```python
from build123d import *

# Parameters (mm, degrees)
PAD_DEPTH    = 25
POCKET_DEPTH = 5
FILLET_R     = 1


with BuildPart() as part:
    # Sketch → Pad (new body)
    with BuildSketch(Plane.XY):
        with BuildLine():
            Line((-6.8, 40), (-6.8, 0))
            Line((-6.8, 0), (-5.8, 0))
            ThreePointArc((-5.8, 0), (-4.679209, 3.420545), (-4.3, 7))
            Line((-4.3, 7), (-4.3, 37))
            ThreePointArc((-2.5, 37), (-3.4, 37.9), (-4.3, 37))
            Line((-2.5, 37), (-2.5, 6.999997))
            ThreePointArc((-2.5, 6.999997), (-1.632155, 3.363514), (0, 0))
            Line((0, 0), (0, 40))
            ThreePointArc((0, 40), (-3.4, 43.4), (-6.8, 40))
        make_face()
    extrude(amount=PAD_DEPTH)

    # Sketch001 → Pocket (cut)
    with BuildSketch(Plane(origin=(-7.5, 0, 0), x_dir=(0, -1, 0), z_dir=(-1, 0, 0))):
        with BuildLine():
            ThreePointArc((-12.608682, 0), (-0.108682, 12.5), (-12.608682, 25))
            Line((-12.608682, 25), (7.391318, 25))
            Line((7.391318, 25), (7.391318, 0))
            Line((7.391318, 0), (-12.608682, 0))
        make_face()
    extrude(amount=-POCKET_DEPTH, mode=Mode.SUBTRACT)

    # Fillet
    fillet_edges = [part.edges().sort_by_distance(p)[0] for p in [
        (-6.8, 26.304341, 0),
        (-6.8, 0.108682, 12.5),
        (-6.8, 26.304341, 25),
        (-6.8, 40, 12.5),
    ]]
    fillet(fillet_edges, radius=FILLET_R)


solid = part.part
```
Input: part model. Units: mm. Frame: model coordinates. A direction names the side the tool comes from. Round coordinates to 2 decimals unless told otherwise and drop trailing zeros. Loops run counter-clockwise (first coordinate to the right, second up) from the corner with the lowest first, then second, coordinate; pieces in that order, holes last.
1) Set-up query: faces 5 (the cylindrical face through (-5.56, 0.96, 7.97)), 6 (the flat face through (-4.3, 22, 12)), 7 (the cylindrical face through (-6.515, 26.496, 24.699)). Return all of +Z, -Z, +X, -X, +Y, -Y with unobstructed straight access to the full face (end or side cutting, diameter ignored); none if empty.
Ans:
face 5: -X, -Y
face 6: +Z, -Z, -Y
face 7: +Z, -X, +Y, -Y
2) Pull-direction query (X, two-part tool) for faces 1 (the cylindrical face through (-1.65, 3.41, 12.32)), 2 (the flat face through (-2.5, 22, 12)), 3 (the flat face through (0, 20, 12)), 4 (the flat face through (-6.8, 21, 12)); classes: released by +X, released by -X, zero draft, split by the parting line, or undercut.
Ans:
face 1: undercut
face 2: undercut
face 3: released by +X
face 4: released by -X
3) Section query C-C on x = -3.4. Return the cut outline in (y, z).
Ans:
outline: (37.9, 0) - (42.4, 0) arc R1 ccw to (43.4, 1) - (43.4, 24) arc R1 ccw to (42.4, 25) - (37.9, 25) - close
4) Pin query (flat end, axial travel): pin 1 (2 mm diameter, centred on x = -5, z = 12.5, fed in from +Y); pin 2 (1.5 mm diameter, centred on x = -5.5, z = 18, fed in from +Y). Return the tip coordinate at first contact, or that it passes through.
Ans:
pin 1: stops at y = 43.35
pin 2: stops at y = 43.12
5) Section query A-A on y = 18.5. Return the cut outline in (x, z), plus the area to 3 significant figures.
Ans:
outline: (-6.8, 1) arc R1 ccw to (-5.8, 0) - (-4.3, 0) - (-4.3, 25) - (-5.8, 25) arc R1 ccw to (-6.8, 24) - close; (-2.5, 0) - (-1, 0) arc R1 ccw to (0, 1) - (0, 24) arc R1 ccw to (-1, 25) - (-2.5, 25) - close
area: 124 mm2
6) Material intervals for line 1 (X direction, y = 7.5, z = 21.75); line 2 (X direction, y = 5, z = 19.25); line 3 (Z direction, x = -0.75, y = 37), sorted ascending.
Ans:
line 1: x = -6.8 to -4.3, -2.5 to 0
line 2: x = -6.8 to -4.42, -2.13 to 0
line 3: z = 0.03 to 24.97
7) Section query B-B on z = 12.5. Return the cut outline in (x, y).
Ans:
outline: (-6.8, 1.11) arc R1 ccw to (-5.8, 0.11) - (-5.75, 0.11) arc R17.08 ccw to (-4.3, 7) - (-4.3, 37) arc R0.9 cw to (-2.5, 37) - (-2.5, 7) arc R17.22 ccw to (0, 0) - (0, 40) arc R3.4 ccw to (-6.8, 40) - close
